from build123d import *

# Parameters (mm, degrees)
SKETCH_1_W          = 12.3
SKETCH_1_H          = 11.3
EXTRUDE_1_DEPTH     = 2
SKETCH_2_W          = 1.5
SKETCH_2_H          = 11.3
EXTRUDE_2_DEPTH     = 4.25
SKETCH_5_W          = 9.3
SKETCH_5_H          = 11.5
CUT_EXTRUDE_1_DEPTH = 1
SKETCH_8_W          = 1.6
SKETCH_8_H          = 11.3
EXTRUDE_5_DEPTH     = 0.8
SKETCH_9_W          = 1.6
SKETCH_9_H          = 11.3
EXTRUDE_6_DEPTH     = 0.8
FILLET_7_R          = 0.8
FILLET_8_R          = 0.3


with BuildPart() as part:
    # 스케치1 → 보스-돌출1 (new body)
    with BuildSketch(Plane.XY):
        Rectangle(SKETCH_1_W, SKETCH_1_H)
    extrude(amount=EXTRUDE_1_DEPTH)

    # 스케치2 → 보스-돌출2 (add)
    with BuildSketch(Plane.XY.offset(2)):
        with Locations((-5.4, 0)):
            Rectangle(SKETCH_2_W, SKETCH_2_H)
        with Locations((5.4, 0)):
            Rectangle(SKETCH_2_W, SKETCH_2_H)
    extrude(amount=EXTRUDE_2_DEPTH)

    # 스케치5 → 컷-돌출1 (cut)
    with BuildSketch(Plane.XY.offset(2)):
        Rectangle(SKETCH_5_W, SKETCH_5_H)
    extrude(amount=-CUT_EXTRUDE_1_DEPTH, mode=Mode.SUBTRACT)

    # 스케치8 → 보스-돌출5 (add)
    with BuildSketch(Plane(origin=(-4.65, 0, 0), x_dir=(0, 0, -1), z_dir=(1, 0, 0))):
        with Locations((-5.45, 0)):
            Rectangle(SKETCH_8_W, SKETCH_8_H)
    extrude(amount=EXTRUDE_5_DEPTH)

    # 스케치9 → 보스-돌출6 (add)
    with BuildSketch(Plane.ZY.offset(-4.65)):
        with Locations((5.45, 0)):
            Rectangle(SKETCH_9_W, SKETCH_9_H)
    extrude(amount=EXTRUDE_6_DEPTH)

    # 필렛7
    fillet_7_edges = [part.edges().sort_by_distance(p)[0] for p in [
        (3.85, 0, 6.25),
        (-3.85, 0, 6.25),
        (3.85, 0, 4.65),
        (-3.85, 0, 4.65),
    ]]
    fillet(fillet_7_edges, radius=FILLET_7_R - 0.0001)  # a hair under: the kernel refuses the full size

    # 필렛8
    fillet_8_edges = [part.edges().sort_by_distance(p)[0] for p in [
        (4.65, 0, 1),
        (-4.65, 0, 1),
    ]]
    fillet(fillet_8_edges, radius=FILLET_8_R)


solid = part.part
The listing builds one solid part. Answer for the finished solid, in the listing's coordinates (mm). A direction names the side the tool comes from. Give positions to 0.01 mm unless a question says otherwise; leave off trailing zeros. Order: outer loops, then holes, each group sorted by start corner. A loop starts at its lowest first (then second) coordinate and runs counter-clockwise, first axis right, second up. Notation, with made-up numbers: (24, 81.5) - (47, 81.5) arc R14 cw to (47, 87.5) - close; hole circle Ø8 at (-14, 65.5). An arc over 180 degrees is marked (long way). Use one line per item in the form item = value.
1) Find section B-B on x = 4. Determine the outline of the cut face in (y, z), and give its area (3 significant figures).
Verdict:
outline = (-5.65, 0) - (5.65, 0) - (5.65, 1) - (-5.65, 1) - close; (-5.65, 4.98) - (5.65, 4.98) - (5.65, 5.92) - (-5.65, 5.92) - close
area = 21.8 mm^2
2) Find section D-D on x = -0.25. Determine the outline of the cut face in (y, z), and give its area (3 significant figures).
Verdict:
outline = (-5.65, 0) - (5.65, 0) - (5.65, 1) - (-5.65, 1) - close
area = 11.3 mm^2
3) Each of these flat-tipped pins is pushed along its axis until it touches: pin 1 (6 mm diameter, centred on x = 0, y = -4.5, fed in from -Z); pin 2 (5 mm diameter, centred on x = 0, y = -0.5, fed in from +Z). Where does it stop, or does it pass through?
Verdict:
pin_1 = 0
pin_2 = 1
4) For faces 1 (the flat face through (-6.15, 0, 3)), 2 (the flat face through (-4.65, 0, 3)), determine the directions among +Z, -Z, +X, -X, +Y, -Y from which every point of the face is accessible in a straight line to the end or side of a thin tool.
Verdict:
face_1 = +Z, -Z, -X, +Y, -Y
face_2 = +Y, -Y
5) Consider probe 1 along X at (y, z) = (0, 1.25); probe 2 along Z at (x, y) = (0, 3.5); probe 3 along X at (y, z) = (0, 5.5). Determine where each line is inside the solid, lowest interval first. Write a range as [from, to].
Verdict:
probe_1 = [-6.15, -4.65], [4.65, 6.15]
probe_2 = [0, 1]
probe_3 = [-6.15, -3.85], [3.85, 6.15]
6) Find section A-A on z = 2.5. Determine the outline of the cut face in (x, y), and give its area (3 significant figures).
Verdict:
outline = (-6.15, -5.65) - (-4.65, -5.65) - (-4.65, 5.65) - (-6.15, 5.65) - close; (4.65, -5.65) - (6.15, -5.65) - (6.15, 5.65) - (4.65, 5.65) - close
area = 33.9 mm^2
7) The mould has two halves that part along X. Classify faces 3 (the flat face through (4.65, 0, 3)), 4 (the flat face through (0, 0, 1)), 5 (the flat face through (0.1, 5.65, 0.3)), 6 (the flat face through (6.15, 0, 3)): released by +X, released by -X, zero draft, split by the parting line, or undercut.
Verdict:
face_3 = undercut
face_4 = undercut
face_5 = zero draft
face_6 = released by +X
